from build123d import *

# Parameters (mm, degrees)
CROQUIS1_W              = 72.136
CROQUIS1_H              = 38.1
SALIENTE_EXTRUIR1_DEPTH = 96.52
VACIADO1_T              = -4
CROQUIS2_W              = 2.032
CROQUIS2_H              = 30.226
SALIENTE_EXTRUIR2_DEPTH = 96.52
CROQUIS3_W              = 16
CROQUIS3_H              = 4
SALIENTE_EXTRUIR3_DEPTH = 4


with BuildPart() as part:
    # Croquis1 → Saliente-Extruir1 (new body)
    with BuildSketch(Plane.XY):
        Rectangle(CROQUIS1_W, CROQUIS1_H)
    extrude(amount=SALIENTE_EXTRUIR1_DEPTH)

    # Vaciado1
    vaciado1_openings = [part.faces().sort_by_distance(p)[0] for p in [
        (0, 19.05, 48.26),
    ]]
    offset(amount=VACIADO1_T, openings=vaciado1_openings, kind=Kind.INTERSECTION)

    # Croquis2 → Saliente-Extruir2 (add)
    with BuildSketch(Plane.XY.offset(96.52)):
        with Locations((-37.084, 0.127)):
            Rectangle(CROQUIS2_W, CROQUIS2_H)
        with Locations((37.084, 0.127)):
            Rectangle(CROQUIS2_W, CROQUIS2_H)
    extrude(amount=-SALIENTE_EXTRUIR2_DEPTH)

    # Croquis3 → Saliente-Extruir3 (add)
    with BuildSketch(Plane.XY.offset(96.52)):
        with Locations((-1.770271924, -13.05)):
            Rectangle(CROQUIS3_W, CROQUIS3_H)
    extrude(amount=SALIENTE_EXTRUIR3_DEPTH)


solid = part.part
Could you check a few things on this model? Use its own coordinates, in mm. A direction names the side the tool comes from. Round coordinates to 2 decimals unless told otherwise and drop trailing zeros. Order: outer loops, then holes, each group sorted by start corner. A loop starts at its lowest first (then second) coordinate and runs counter-clockwise, first axis right, second up.
(1) I'm going to push flat-ended pins straight in: pin 1 (19 mm diameter, centred on x = -16, y = -2.5, fed in from +Z); pin 2 (1.1 mm diameter, centred on y = 17.5, z = 48, fed in from -X); pin 3 (3 mm diameter, centred on y = -12.5, z = 99.5, fed in from -X); pin 4 (10 mm diameter, centred on x = -14, y = 3.5, fed in from -Z). Where does each tip first touch, or does it pass through?
Response values:
pin 1: stops at z = 96.52
pin 2: stops at x = -36.07
pin 3: stops at x = -9.77
pin 4: stops at z = 0
(2) Imagine slicing it at A-A (y = 9.5). Write out the boundary of the cut face in (x, z).
Response values:
outline: (-38.1, 0) - (38.1, 0) - (38.1, 96.52) - (-38.1, 96.52) - close; hole (-32.07, 4) - (32.07, 4) - (32.07, 92.52) - (-32.07, 92.52) - close
(3) Please list where these lines run through material, in increasing order: line 1 along Z through (x, y) = (-19, 1.5); line 2 along X through (y, z) = (17.5, 61); line 3 along X through (y, z) = (13, 79).
Response values:
line 1: z = 0 to 4, 92.52 to 96.52
line 2: x = -36.07 to -32.07, 32.07 to 36.07
line 3: x = -38.1 to -32.07, 32.07 to 38.1
(4) If we mould it in two halves opening along Z, with no side actions, what happens to faces 1 (the flat face through (-38.1, 0, 49)), 2 (the flat face through (-2, -13, 100.52)), 3 (the flat face through (32.068, 2, 48))? For each: released by +Z, released by -Z, zero draft, split by the parting line, or undercut.
Response values:
face 1: zero draft
face 2: released by +Z
face 3: undercut
(5) Imagine slicing it at D-D (x = -26.5). Write out the boundary of the cut face in (y, z), plus the area to 3 significant figures.
Response values:
outline: (-19.05, 0) - (19.05, 0) - (19.05, 4) - (-15.05, 4) - (-15.05, 92.52) - (19.05, 92.52) - (19.05, 96.52) - (-19.05, 96.52) - close
area: 659 mm2
(6) Imagine slicing it at C-C (z = 16.5). Write out the boundary of the cut face in (x, y).
Response values:
outline: (-38.1, -14.99) - (-36.07, -14.99) - (-36.07, -19.05) - (36.07, -19.05) - (36.07, -14.99) - (38.1, -14.99) - (38.1, 15.24) - (36.07, 15.24) - (36.07, 19.05) - (32.07, 19.05) - (32.07, -15.05) - (-32.07, -15.05) - (-32.07, 19.05) - (-36.07, 19.05) - (-36.07, 15.24) - (-38.1, 15.24) - close
(7) Imagine slicing it at B-B (x = -6.5). Write out the boundary of the cut face in (y, z), plus the area to 3 significant figures.
Response values:
outline: (-19.05, 0) - (19.05, 0) - (19.05, 4) - (-15.05, 4) - (-15.05, 92.52) - (19.05, 92.52) - (19.05, 96.52) - (-11.05, 96.52) - (-11.05, 100.52) - (-15.05, 100.52) - (-15.05, 96.52) - (-19.05, 96.52) - close
area: 675 mm2
(8) Which directions (+Z, -Z, +X, -X, +Y, -Y) give clear straight access to the entire face, cutting with the end or side of a thin tool? Please do faces 4 (the flat face through (-37, 15.24, 49)), 5 (the flat face through (-36.068, -17, 48)), 6 (the flat face through (0, 2, 4)), 7 (the flat face through (-9.77, -13, 98)), 8 (the flat face through (-2, -11.05, 98)).
Response values:
face 4: +Z, -Z, -X, +Y
face 5: +Z, -Z, -X, -Y
face 6: +Y
face 7: +Z, -X, +Y, -Y
face 8: +Z, +X, -X, +Y
